Design review of the part built by this model. Coordinates are the model's own, in mm. Coordinates: 2 decimals unless noted, no trailing zeros. Loops run counter-clockwise (first coordinate to the right, second up) from the corner with the lowest first, then second, coordinate; pieces in that order, holes last. Notation, with made-up numbers: (-25, 30) -> (-4, 30) arc R20 cw to (-4, 63) -> close; hole circle Ø2 at (65.25, 36). An arc over 180 degrees is marked (long way). Answer as a JSON object with one key per item and string values.
```python
from build123d import *

# Parameters (mm, degrees)
BOSS_EXTRUDE1_DEPTH = 1.5
FILLET1_R           = 1.5875
SKETCH2_W           = 3
SKETCH2_H           = 6.35
BOSS_EXTRUDE2_DEPTH = 3
FILLET2_R           = 0.79375


with BuildPart() as part:
    # Sketch1 → Boss-Extrude1 (new, symmetric)
    with BuildSketch(Plane(origin=(0, 0, 0), x_dir=(1, 0, 0), z_dir=(0, 1, 0))):
        Polygon((25.4, 12.7), (9.525, 12.7), (9.525, -12.7), (25.4, -12.7), (25.4, -25.4), (9.525, -25.4), (0, -25.4), (-9.525, -25.4), (-25.4, -25.4), (-25.4, -12.7), (-9.525, -12.7), (-9.525, 12.7), (-25.4, 12.7), (-25.4, 25.4), (-11.1125, 25.4), (-11.1125, 22.225), (11.1125, 22.225), (11.1125, 25.4), (25.4, 25.4), align=None)
    extrude(amount=BOSS_EXTRUDE1_DEPTH, both=True)

    # Fillet1
    fillet1_edges = [part.edges().sort_by_distance(p)[0] for p in [
        (25.4, 0, -12.7),
        (9.525, 0, -12.7),
        (9.525, 0, 12.7),
        (25.4, 0, 12.7),
        (25.4, 0, 25.4),
        (-25.4, 0, 12.7),
        (-9.525, 0, 12.7),
        (-9.525, 0, -12.7),
        (-25.4, 0, -12.7),
        (-25.4, 0, -25.4),
        (-25.4, 0, 25.4),
        (25.4, 0, -25.4),
        (-11.1125, 0, -25.4),
        (-11.1125, 0, -22.225),
        (11.1125, 0, -22.225),
        (11.1125, 0, -25.4),
    ]]
    fillet(fillet1_edges, radius=FILLET1_R - 0.0001)  # a hair under: the kernel refuses the full size

    # Sketch2 → Boss-Extrude2 (add)
    with BuildSketch(Plane(origin=(0, 1.5, 0), x_dir=(1, 0, 0), z_dir=(0, 1, 0))):
        with Locations((-26.9, 19.05)):
            Rectangle(SKETCH2_W, SKETCH2_H)
        with Locations((26.9, 19.05)):
            Rectangle(SKETCH2_W, SKETCH2_H)
        with Locations((26.9, -19.05)):
            Rectangle(SKETCH2_W, SKETCH2_H)
        with Locations((-26.9, -19.05)):
            Rectangle(SKETCH2_W, SKETCH2_H)
    extrude(amount=-BOSS_EXTRUDE2_DEPTH)

    # Fillet2
    fillet2_edges = [part.edges().sort_by_distance(p)[0] for p in [
        (-28.4, 0, 22.225),
        (-28.4, 0, 15.875),
        (28.4, 0, 15.875),
        (28.4, 0, 22.225),
        (28.4, 0, -22.225),
        (28.4, 0, -15.875),
        (-28.4, 0, -15.875),
        (-28.4, 0, -22.225),
    ]]
    fillet(fillet2_edges, radius=FILLET2_R)


solid = part.part
```
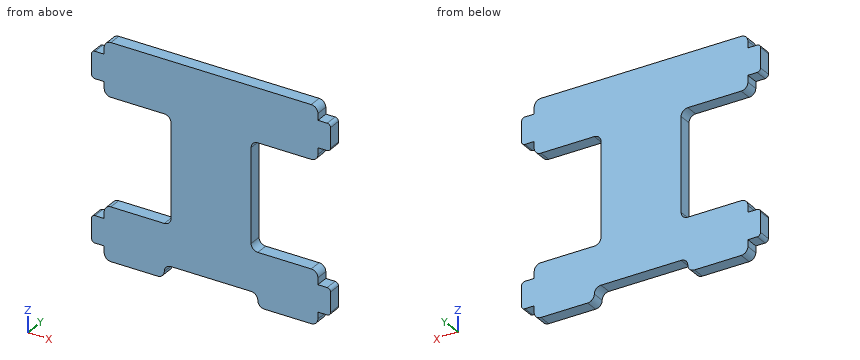
1) Add section C-C, the plane x = 1. Give the boundary of the cut face in (y, z) (3 decimals), and give its area (3 significant figures).
Completed:
{"outline": "(-1.5, -22.225) -> (1.5, -22.225) -> (1.5, 25.4) -> (-1.5, 25.4) -> close", "area": "143 mm²"}
2) Add section A-A, the plane x = -10.5. Give the boundary of the cut face in (y, z).
Completed:
{"outline": "(-1.5, -22.56) -> (1.5, -22.56) -> (1.5, -12.58) -> (-1.5, -12.58) -> close; (-1.5, 12.58) -> (1.5, 12.58) -> (1.5, 25.4) -> (-1.5, 25.4) -> close"}
3) Add section B-B, the plane z = 15. Give the boundary of the cut face in (x, y).
Completed:
{"outline": "(-25.4, -1.5) -> (25.4, -1.5) -> (25.4, 1.5) -> (-25.4, 1.5) -> close"}
4) Clearance check with flat-ended pins moving along their axes: pin 1 Ø0.8 at (y, z) = (0, -23) entering from +X; pin 2 Ø1 at (y, z) = (0, -12.5) entering from -X; pin 3 Ø1.1 at (x, y) = (-26.5, 0) entering from +Z (3 decimals). State where each tip first meets the part, or that it passes through.
Completed:
{"pin 1": "x = 25.4", "pin 2": "x = -24.74", "pin 3": "z = 22.225"}
5) Wall thickness on probe 1 along Z at (x, y) = (-19, 1.35); probe 2 along X at (y, z) = (-0.8, 23.5); probe 3 along X at (y, z) = (0.05, 10.5) (3 decimals): over which ranges is each line inside the solid? List them lowest first.
Completed:
{"probe 1": "-25.4 to -12.7, 12.7 to 25.4", "probe 2": "-25.4 to 25.4", "probe 3": "-9.525 to 9.525"}
